Part model, mm, in its own coordinate system. A direction names the side the tool comes from. Give positions to 0.01 mm unless a question says otherwise; leave off trailing zeros. Order: outer loops, then holes, each group sorted by start corner. A loop starts at its lowest first (then second) coordinate and runs counter-clockwise, first axis right, second up. Notation, with made-up numbers: M -29,-11.5 L -14,-11.5 A10 ccw -14,-2.5 Z; hole C 84.5,-7 d5. An arc over 180 degrees is marked long. Return JSON: item names as keys, results as strings.
from build123d import *

# Parameters (mm, degrees)
F0_W     = 200
F0_H     = 18
F1_DEPTH = 2
F2_W     = 200
F2_H     = 2.4
F3_DEPTH = 40
F5_DEPTH = 18
F6_W     = 4
F6_H     = 40
F7_DEPTH = 22.801


with BuildPart() as f1:
    # F0 (on Top) → F1 (new body)
    with BuildSketch(Plane.XY):
        with Locations((100, 9)):
            Rectangle(F0_W, F0_H)
    extrude(amount=F1_DEPTH)

    # F2 (on face) → F3 (join)
    with BuildSketch(Plane(origin=(0, 0, 0), x_dir=(1, 0, 0), z_dir=(0, 0, -1))):
        with Locations((100, 1.2)):
            Rectangle(F2_W, F2_H)
        with Locations((100, -19.2)):
            Rectangle(F2_W, F2_H)
    extrude(amount=-F3_DEPTH)

    # F4 (on face) → F5 (join, through all)
    with BuildSketch(Plane.XZ.offset(-18)):
        Polygon((2, 25), (0, 2), (4, 2), align=None)
        Polygon((10, 2), (8, 25), (6, 2), align=None)
        Polygon((16, 2), (14, 25), (12, 2), align=None)
        Polygon((22, 2), (20, 25), (18, 2), align=None)
        Polygon((28, 2), (26, 25), (24, 2), align=None)
        Polygon((34, 2), (32, 25), (30, 2), align=None)
        Polygon((40, 2), (38, 25), (36, 2), align=None)
        Polygon((46, 2), (44, 25), (42, 2), align=None)
        Polygon((52, 2), (50, 25), (48, 2), align=None)
        Polygon((58, 2), (56, 25), (54, 2), align=None)
        Polygon((64, 2), (62, 25), (60, 2), align=None)
        Polygon((70, 2), (68, 25), (66, 2), align=None)
        Polygon((76, 2), (74, 25), (72, 2), align=None)
        Polygon((82, 2), (80, 25), (78, 2), align=None)
        Polygon((88, 2), (86, 25), (84, 2), align=None)
        Polygon((94, 2), (92, 25), (90, 2), align=None)
        Polygon((100, 2), (98, 25), (96, 2), align=None)
        Polygon((106, 2), (104, 25), (102, 2), align=None)
        Polygon((112, 2), (110, 25), (108, 2), align=None)
        Polygon((118, 2), (116, 25), (114, 2), align=None)
        Polygon((124, 2), (122, 25), (120, 2), align=None)
        Polygon((130, 2), (128, 25), (126, 2), align=None)
        Polygon((136, 2), (134, 25), (132, 2), align=None)
        Polygon((142, 2), (140, 25), (138, 2), align=None)
        Polygon((148, 2), (146, 25), (144, 2), align=None)
        Polygon((154, 2), (152, 25), (150, 2), align=None)
        Polygon((160, 2), (158, 25), (156, 2), align=None)
        Polygon((166, 2), (164, 25), (162, 2), align=None)
        Polygon((172, 2), (170, 25), (168, 2), align=None)
        Polygon((178, 2), (176, 25), (174, 2), align=None)
        Polygon((184, 2), (182, 25), (180, 2), align=None)
        Polygon((190, 2), (188, 25), (186, 2), align=None)
        Polygon((196, 2), (194, 25), (192, 2), align=None)
    extrude(amount=F5_DEPTH)

    # F6 (on face) → F7 (cut, through all)
    with BuildSketch(Plane(origin=(0, 20.4, 0), x_dir=(-1, 0, 0), z_dir=(0, 1, 0))):
        with Locations((-198, 20)):
            Rectangle(F6_W, F6_H)
    extrude(amount=-F7_DEPTH, mode=Mode.SUBTRACT)


solid = f1.part
Q1. Probe line 1 along Y through (x, z) = (122, 37); line 2 along Z through (x, y) = (185.5, 3.5). List the from-to ranges inside material, lowest first.
Established:
{"line 1": "y = -2.4 to 0, 18 to 20.4", "line 2": "z = 0 to 2"}
Q2. Pin check, flat tips, straight feed: pin 1 (12 mm diameter, centred on y = 14.5, z = 6.5, fed in from +X); pin 2 (3 mm diameter, centred on y = 13.5, z = 24, fed in from -X); pin 3 (1 mm diameter, centred on x = 131, y = 7.5, fed in from +Z). Stop position of each tip, or through.
Established:
{"pin 1": "stops at x = 196", "pin 2": "stops at x = 1.78", "pin 3": "stops at z = 2"}
Q3. 3-axis set-ups, long thin cutter, end or side, ignore diameter. For faces 4 (the flat face through (139.014, 9.126, 13.661)), 5 (the flat face through (97, 20.4, 20)): which of +Z, -Z, +X, -X, +Y, -Y reach the whole face in a straight line?
Established:
{"face 4": "+Z", "face 5": "+Z, -Z, +X, -X, +Y"}
Q4. Two-plate mould, pull along X, no slides. Class faces 1 (the flat face through (195.014, 9.126, 13.339)), 2 (the flat face through (15.014, 9.126, 13.339)), 3 (the flat face through (97, 9, 0)): +X half, -X half, draft (parallel to the pull), parting line (faces both ways), or undercut.
Established:
{"face 1": "+X half", "face 2": "undercut", "face 3": "draft"}
Q5. Band-saw the part on B-B (z = 21). Give the number of separate pieces and of enclosed holes in the cut face, then the cut area to 3 significant figures.
Established:
{"separate pieces": "1", "enclosed holes": "32", "area": "1,350 mm²"}
Q6. Band-saw the part on A-A (z = 37.5). Give the cut face in (x, y).
Established:
{"outline": "M 0,-2.4 L 196,-2.4 L 196,0 L 0,0 Z; M 0,18 L 196,18 L 196,20.4 L 0,20.4 Z"}
